For this review, take the finished solid that the model builds, in its own axes (mm). Face numbers are marked on the shaded views. A direction names the side the tool comes from. Coordinates: 2 decimals unless noted, no trailing zeros. Write each loop counter-clockwise with the first axis right and the second up, starting at its lowest first coordinate (ties: lowest second). Pieces come first, ordered by that corner, then holes. Notation, with made-up numbers: (72, 45.25) - (124, 45.25) arc R31 cw to (124, 83.25) - close; hole circle Ø11 at (-17.5, -37). An arc over 180 degrees is marked (long way). Write each question's results on one line, items separated by ' | '.
from build123d import *

# Parameters (mm, degrees)
SKETCH1_R                = 24.511
BOSS_EXTRUDE1_DEPTH      = 508
SKETCH2_R                = 7.62
BOSS_EXTRUDE2_DEPTH      = 25.4
BOSS_EXTRUDE2_DEPTH_BACK = 533.4


with BuildPart() as part:
    # Sketch1 → Boss-Extrude1 (new body)
    with BuildSketch(Plane(origin=(0, 0, 0), x_dir=(1, 0, 0), z_dir=(0, 1, 0))):
        Circle(SKETCH1_R)
    extrude(amount=BOSS_EXTRUDE1_DEPTH)

    # Sketch2 → Boss-Extrude2 (add, two sides)
    with BuildSketch(Plane.XZ) as boss_extrude2_sk:
        Circle(SKETCH2_R)
    extrude(amount=BOSS_EXTRUDE2_DEPTH)
    extrude(boss_extrude2_sk.sketch, amount=-BOSS_EXTRUDE2_DEPTH_BACK)


solid = part.part
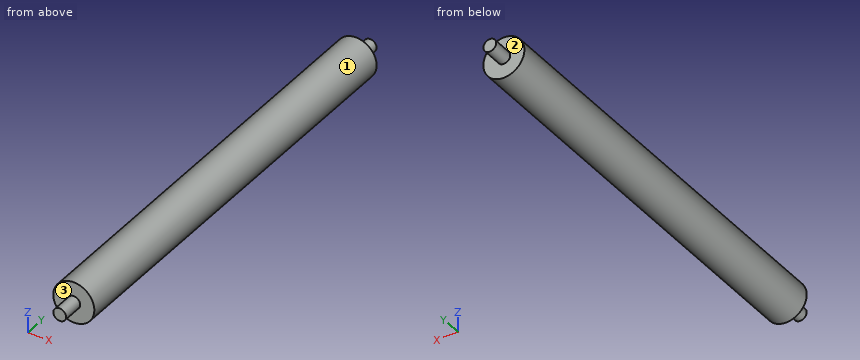
Q1. Take a section at B-B on x = 0. State the section outline as (y, z) points, plus the area to 3 significant figures.
Results found:
outline: (-25.4, -7.62) - (0, -7.62) - (0, -24.51) - (508, -24.51) - (508, -7.62) - (533.4, -7.62) - (533.4, 7.62) - (508, 7.62) - (508, 24.51) - (0, 24.51) - (0, 7.62) - (-25.4, 7.62) - close | area: 25,700 mm2
Q2. Take a section at C-C on y = 151. State the section outline as (x, z) points, plus the area to 3 significant figures.
Results found:
outline: circle Ø49.02 at (0, 0) | area: 1,890 mm2
Q3. Wall thickness on line 1 along Y through (x, z) = (-11, -8); line 2 along Z through (x, y) = (-0.5, 64); line 3 along Z through (x, y) = (-3.5, 328): over which ranges is each line inside the solid? List them lowest first. Write a range as from..to.
Results found:
line 1: 0..508 | line 2: -24.51..24.51 | line 3: -24.26..24.26
Q4. For the marked faces 1, 2 and 3, list the 3-axis set-ups (+Z, -Z, +X, -X, +Y, -Y) from which the entire face can be reached by the end or side of a thin tool; tool diameter is ignored.
Results found:
face 1: +Y, -Y | face 2: +Y | face 3: -Y
Q5. Take a section at A-A on z = 0. State the section outline as (x, y) points, plus the area to 3 significant figures.
Results found:
outline: (-24.51, 0) - (-7.62, 0) - (-7.62, -25.4) - (7.62, -25.4) - (7.62, 0) - (24.51, 0) - (24.51, 508) - (7.62, 508) - (7.62, 533.4) - (-7.62, 533.4) - (-7.62, 508) - (-24.51, 508) - close | area: 25,700 mm2
Q6. For pin 1 (1.5 mm diameter, centred on y = 286, z = 15, fed in from -X); pin 2 (1 mm diameter, centred on x = -16, y = 153, fed in from -Z); pin 3 (2 mm diameter, centred on y = 324, z = 13.5, fed in from -X); pin 4 (8 mm diameter, centred on x = 10.5, z = -4, fed in from +Y), all flat-tipped, find the tip position at first contact; note any pin that passes through.
Results found:
pin 1: x = -19.94 | pin 2: z = -18.99 | pin 3: x = -21.08 | pin 4: y = 533.4
